Build history of the part. All positions in model axes, mm. Round coordinates to 2 decimals unless told otherwise and drop trailing zeros. Write each loop counter-clockwise with the first axis right and the second up, starting at its lowest first coordinate (ties: lowest second). Pieces come first, ordered by that corner, then holes. Notation, with made-up numbers: M -33.5,29.5 L -26.5,29.5 A18 ccw -26.5,60.5 Z; hole C -30,-34 d9. An arc over 180 degrees is marked long. Use a Markdown table: item, result.
from build123d import *

# Parameters (mm, degrees)
FILLET_R     = 0.2
POCKET_DEPTH = 0.5
FILLET001_R  = 0.05


with BuildPart() as part:
    # Sketch → Revolution (revolve)
    with BuildSketch(Plane.XY):
        Polygon((0, 0), (0, 8.8), (1.55, 8.8), (1.55, 7.5), (1, 7.5), (1, 0), align=None)
    revolve(axis=Axis((0, 0, 0), (0, 1, 0)))

    # Fillet
    fillet_edges = [part.edges().sort_by_distance(p)[0] for p in [
        (-1.55, 8.8, 0),
        (-1.55, 7.5, 0),
    ]]
    fillet(fillet_edges, radius=FILLET_R)

    # Sketch001 (on Face1 of Fillet) → Pocket (cut)
    with BuildSketch(Plane(origin=(0, 8.8, 0), x_dir=(-1, 0, 0), z_dir=(0, 1, 0))):
        Polygon((0, 1), (0.3, 1), (0.3, 0.3), (1, 0.3), (1, -0.3), (0.3, -0.3), (0.3, -1), (0, -1), align=None)
    pocket = extrude(amount=-POCKET_DEPTH, mode=Mode.SUBTRACT)

    # Mirrored: Pocket across Sketch001 V_Axis
    add(pocket.mirror(Plane(origin=(0, 8.8, 0), x_dir=(0, 1, 0), z_dir=(-1, 0, 0))), mode=Mode.SUBTRACT)

    # Fillet001
    fillet001_edges = [part.edges().sort_by_distance(p)[0] for p in [
        (-0.65, 8.8, 0.3),
        (-1, 8.8, 0),
        (-0.65, 8.8, -0.3),
        (-0.3, 8.8, -0.65),
        (-0.15, 8.8, -1),
        (0.15, 8.8, -1),
        (0.3, 8.8, -0.65),
        (0.65, 8.8, -0.3),
        (0.65, 8.8, 0.3),
        (1, 8.8, 0),
        (0.3, 8.8, 0.65),
        (-0.3, 8.8, 0.65),
        (-0.15, 8.8, 1),
        (0.15, 8.8, 1),
    ]]
    fillet(fillet001_edges, radius=FILLET001_R)


solid = part.part
Q1. Two-plate mould, pull along X, no slides. Class faces 1 (the flat face through (0, 8.3, 0)), 2 (the cylindrical face through (0, 4, 1)), 3 (the flat face through (0, 0, 0)): +X half, -X half, draft (parallel to the pull), parting line (faces both ways), or undercut.
Response values:
| item | result |
|---|---|
| face 1 | undercut |
| face 2 | parting line |
| face 3 | draft |
Q2. Cut at C-C on y = 2.25. Give the cut face in (x, z).
Response values:
| item | result |
|---|---|
| outline | C 0,0 d2 |
Q3. Cut at A-A on z = 0. Give the cut face in (x, y), and give its area (3 significant figures).
Response values:
| item | result |
|---|---|
| outline | M -1.55,7.7 A0.2 ccw -1.35,7.5 L -1,7.5 L -1,0 L 1,0 L 1,7.5 L 1.35,7.5 A0.2 ccw 1.55,7.7 L 1.55,8.6 A0.2 ccw 1.35,8.8 L 1.05,8.8 A0.05 ccw 1,8.75 L 1,8.3 L -1,8.3 L -1,8.75 A0.05 ccw -1.05,8.8 L -1.35,8.8 A0.2 ccw -1.55,8.6 Z |
| area | 18.0 mm2 |
Q4. Drop flat-ended pins along their axis: P1, Ø0.5, axis at x = -1, y = 8.5, coming from the -Z side; P2, Ø0.5, axis at x = 1, y = 8.5, coming from the +Z side; P3, Ø0.5, axis at x = 0.5, y = 8.5, coming from the -Z side. Give the stop position or say it passes through.
Response values:
| item | result |
|---|---|
| P1 | stops at z = -1.36 |
| P2 | stops at z = 1.36 |
| P3 | stops at z = -1.53 |
Q5. Drill centre lines: L1, parallel to Y at x = 0.7, z = 0.9; L2, parallel to Y at x = 0.6, z = -0.25; L3, parallel to Z at x = 0, y = 2.75. Where is each one in solid material? Low to high.
Response values:
| item | result |
|---|---|
| L1 | y = 7.5 to 8.8 |
| L2 | y = 0 to 8.3 |
| L3 | z = -1 to 1 |
Q6. Cut at B-B on x = 0. Give the cut face in (y, z).
Response values:
| item | result |
|---|---|
| outline | M 0,-1 L 7.5,-1 L 7.5,-1.35 A0.2 ccw 7.7,-1.55 L 8.6,-1.55 A0.2 ccw 8.8,-1.35 L 8.8,-1.05 A0.05 ccw 8.75,-1 L 8.3,-1 L 8.3,1 L 8.75,1 A0.05 ccw 8.8,1.05 L 8.8,1.35 A0.2 ccw 8.6,1.55 L 7.7,1.55 A0.2 ccw 7.5,1.35 L 7.5,1 L 0,1 Z |
